Drawing for the job (mm, zero at the part's lowest x, y, z). A direction names the side the tool comes from. Coordinates: 2 decimals unless noted, no trailing zeros. Write each loop counter-clockwise with the first axis right and the second up, starting at its lowest first coordinate (ties: lowest second). Pieces come first, ordered by that corner, then holes. Notation, with made-up numbers: M 19,74.5 L 28,74.5 A30 ccw 28,111.5 Z; hole C 16,14 d2. An arc over 180 degrees is marked long. Use a Markdown table: item, result. Add a question column.
Q1. Wall check: L1, parallel to Z at x = 32, y = 1.5; L2, parallel to X at y = 4.25, z = 20; L3, parallel to X at y = 5.5, z = 54.65. Give the ranges that are in metal, low to high. Write a range as from..to.
Q2. Slice it at D-D on z = 48.5. Write the cut outline in (x, y), then the cut area to 3 significant figures.
Q3. Tool access for the marked faces 1 and 2: list every direction of +Z, -Z, +X, -X, +Y, -Y with a clear straight run to the whole face (end or side of a thin tool).
Q4. Slice it at C-C on y = 5. Write the cut outline in (x, z).
Q5. Slice it at A-A on x = 21.5. Write the cut outline in (y, z).
Q6. Mould opens along X. For the marked faces 3, 4 and 5 say: released by +X, released by -X, zero draft, split by the parting line, or undercut.
Q7. Slice it at B-B on z = 33. Write the cut outline in (x, y), then the cut area to 3 significant figures.
Q8. Pin check, flat tips, straight feed: pin 1 Ø2 at (y, z) = (5, 48.5) entering from +X; pin 2 Ø0.8 at (y, z) = (5, 48) entering from -X. Stop position of each tip, or through.
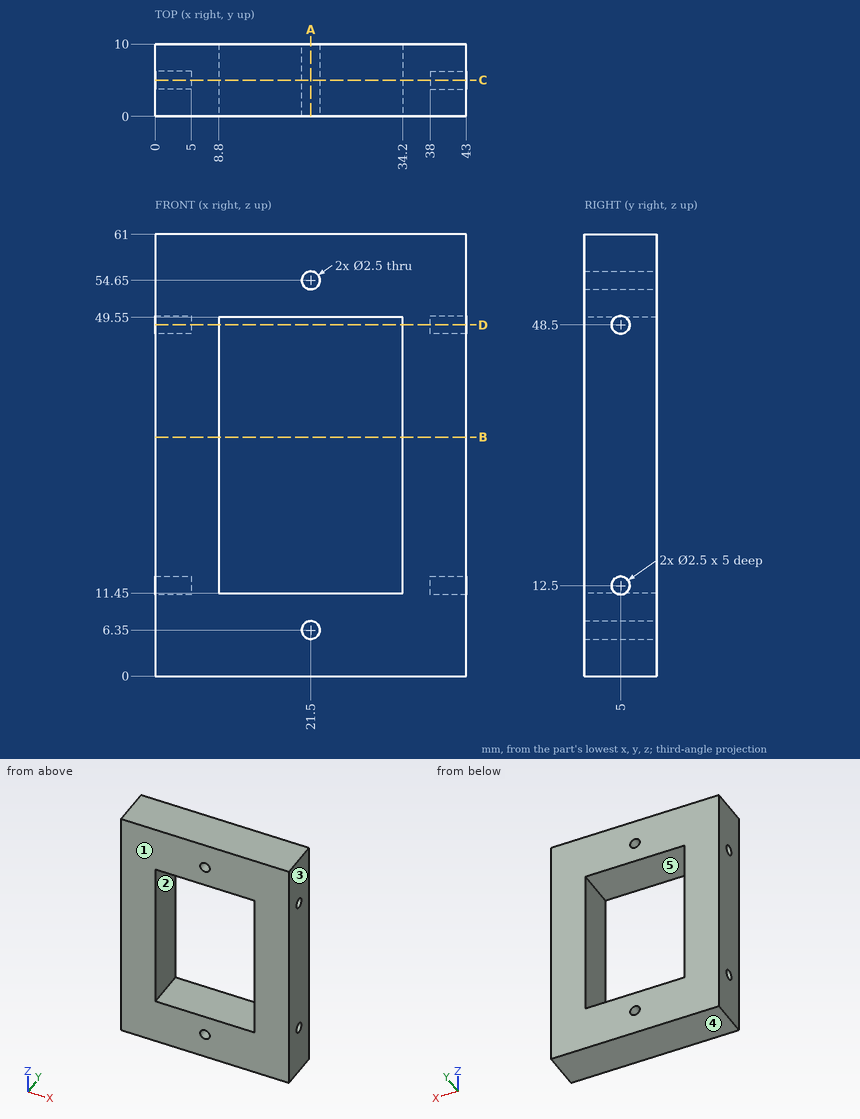
Recorded:
| question | item | result |
|---|---|---|
| 1 | L1 | 0..11.45, 49.55..61 |
| 1 | L2 | 0..8.8, 34.2..43 |
| 1 | L3 | 0..20.25, 22.75..43 |
| 2 | outline | M 0,0 L 8.8,0 L 8.8,10 L 0,10 L 0,6.25 L 5,6.25 L 5,3.75 L 0,3.75 Z; M 34.2,0 L 43,0 L 43,3.75 L 38,3.75 L 38,6.25 L 43,6.25 L 43,10 L 34.2,10 Z |
| 2 | area | 151 mm² |
| 3 | face 1 | +Z, -Z, +X, -X, -Y |
| 3 | face 2 | +Y, -Y |
| 4 | outline | M 0,0 L 43,0 L 43,11.25 L 38,11.25 L 38,13.75 L 43,13.75 L 43,47.25 L 38,47.25 L 38,49.75 L 43,49.75 L 43,61 L 0,61 L 0,49.75 L 5,49.75 L 5,47.25 L 0,47.25 L 0,13.75 L 5,13.75 L 5,11.25 L 0,11.25 Z; hole M 8.8,11.45 L 34.2,11.45 L 34.2,49.55 L 8.8,49.55 Z; hole C 21.5,6.35 d2.5; hole C 21.5,54.65 d2.5 |
| 5 | outline | M 0,0 L 10,0 L 10,5.1 L 0,5.1 Z; M 0,7.6 L 10,7.6 L 10,11.45 L 0,11.45 Z; M 0,49.55 L 10,49.55 L 10,53.4 L 0,53.4 Z; M 0,55.9 L 10,55.9 L 10,61 L 0,61 Z |
| 6 | face 3 | released by +X |
| 6 | face 4 | zero draft |
| 6 | face 5 | undercut |
| 7 | outline | M 0,0 L 8.8,0 L 8.8,10 L 0,10 Z; M 34.2,0 L 43,0 L 43,10 L 34.2,10 Z |
| 7 | area | 176 mm² |
| 8 | pin 1 | x = 38 |
| 8 | pin 2 | x = 5 |
